```python
from build123d import *

# Parameters (mm, degrees)
SKETCH1_W           = 10
SKETCH1_H           = 46.99
SKETCH1_W_2         = 2.049999964
SKETCH1_H_2         = 2.049999964
BOSS_EXTRUDE1_DEPTH = 3.175
SKETCH2_W           = 3.175
SKETCH2_H           = 46.99
BOSS_EXTRUDE2_DEPTH = 3.175


with BuildPart() as part:
    # Sketch1 → Boss-Extrude1 (new body)
    with BuildSketch(Plane(origin=(0, 0, 0), x_dir=(1, 0, 0), z_dir=(0, 1, 0))):
        Rectangle(SKETCH1_W, SKETCH1_H)
        with Locations((0, -18.939243554)):
            Rectangle(SKETCH1_W_2, SKETCH1_H_2, mode=Mode.SUBTRACT)
    extrude(amount=BOSS_EXTRUDE1_DEPTH)

    # Sketch2 → Boss-Extrude2 (add)
    with BuildSketch(Plane(origin=(0, 3.175, 0), x_dir=(1, 0, 0), z_dir=(0, 1, 0))):
        with Locations((-6.5875, 0)):
            Rectangle(SKETCH2_W, SKETCH2_H)
    extrude(amount=-BOSS_EXTRUDE2_DEPTH)


solid = part.part
```
Geometry check sheet. Reference: the model listing, model coordinates, mm. A direction names the side the tool comes from. Give positions to 0.01 mm unless a question says otherwise; leave off trailing zeros. Order: outer loops, then holes, each group sorted by start corner. A loop starts at its lowest first (then second) coordinate and runs counter-clockwise, first axis right, second up. Notation, with made-up numbers: (59, 3.5) - (78, 3.5) arc R32 cw to (78, 40.5) - close; hole circle Ø9 at (88.25, 16.5). An arc over 180 degrees is marked (long way). Write item = value, one per line. Start each with the question number.
1) Section check A-A (x = -0.25). Enter the section's corners in (y, z) (3 decimals).
2) Scan lines: L1, parallel to Z at x = -0.5, y = 0.8 (3 decimals); L2, parallel to X at y = 3.05, z = 18 (3 decimals). Record each from-to range of solid material in increasing order.
3) Draft check along X on faces 1 (the flat face through (0, 2, 17.914)), 2 (the flat face through (-8.175, 2, 0)), 3 (the flat face through (0, 2, 19.964)), 4 (the flat face through (5, 2, 0)). Enter one of: released by +X, released by -X, zero draft, split by the parting line, or undercut.
4) Access from +Z, -Z, +X, -X, +Y, -Y to the whole of each face (thin tool, end or side, straight path). Record for faces 5 (the flat face through (-1.025, 2, 19)), 6 (the flat face through (-2, 2, 23.495)).
Geometry check:
q1.outline = (0, -23.495) - (3.175, -23.495) - (3.175, 17.914) - (0, 17.914) - close; (0, 19.964) - (3.175, 19.964) - (3.175, 23.495) - (0, 23.495) - close
q2.L1 = -23.495 to 17.914, 19.964 to 23.495
q2.L2 = -8.175 to -1.025, 1.025 to 5
q3.face_1 = undercut
q3.face_2 = released by -X
q3.face_3 = undercut
q3.face_4 = released by +X
q4.face_5 = +Y, -Y
q4.face_6 = +Z, +X, -X, +Y, -Y
